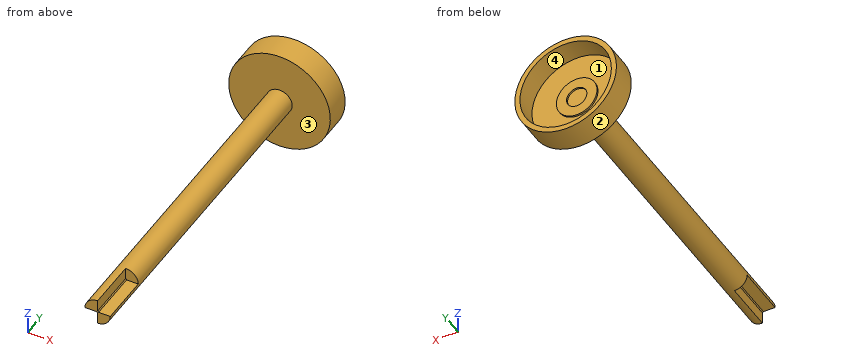
```python
from build123d import *

# Parameters (mm, degrees)
SKETCH1_R           = 10
SKETCH1_R_2         = 9
BOSS_EXTRUDE1_DEPTH = 4.3
BOSS_EXTRUDE2_START = -1
SKETCH1_2_R         = 10
BOSS_EXTRUDE2_DEPTH = 1
SKETCH2_R           = 4
SKETCH2_R_2         = 2
EXTRUDE_THIN1_DEPTH = 0.35
SKETCH3_R           = 2.5
BOSS_EXTRUDE3_DEPTH = 65
CUT_EXTRUDE1_START  = -10
CUT_EXTRUDE1_DEPTH  = 10


with BuildPart() as part:
    # Sketch1 → Boss-Extrude1 (new body)
    with BuildSketch(Plane(origin=(0, 0, 0), x_dir=(1, 0, 0), z_dir=(0, 1, 0))):
        with Locations(Location((0, 0, 0), (0, 0, 90))):
            Circle(SKETCH1_R)
        with Locations(Location((0, 0, 0), (0, 0, 90))):
            Circle(SKETCH1_R_2, mode=Mode.SUBTRACT)
    extrude(amount=BOSS_EXTRUDE1_DEPTH)

    # Sketch1_2 → Boss-Extrude2 (add)
    with BuildSketch(Plane(origin=(0, 0, 0), x_dir=(1, 0, 0), z_dir=(0, 1, 0)).offset(BOSS_EXTRUDE2_START)):
        with Locations(Location((0, 0, 0), (0, 0, 90))):
            Circle(SKETCH1_2_R)
    extrude(amount=BOSS_EXTRUDE2_DEPTH)

    # Sketch2 → Extrude-Thin1 (add)
    with BuildSketch(Plane(origin=(0, 0, 0), x_dir=(1, 0, 0), z_dir=(0, 1, 0))):
        Circle(SKETCH2_R)
        Circle(SKETCH2_R_2, mode=Mode.SUBTRACT)
    extrude(amount=EXTRUDE_THIN1_DEPTH)

    # Sketch3 → Boss-Extrude3 (add)
    with BuildSketch(Plane.XZ.offset(1)):
        with Locations(Location((0, 0, 0), (0, 0, 270))):
            Circle(SKETCH3_R)
    extrude(amount=BOSS_EXTRUDE3_DEPTH)

    # Sketch4 → Cut-Extrude1 (cut)
    with BuildSketch(Plane.XZ.offset(66).offset(CUT_EXTRUDE1_START)):
        with BuildLine():
            Line((-2.5, 0), (-0.194982329, 0))
            ThreePointArc((-0.194982329, 0), (-0.137873327, -0.137873327), (0, -0.194982329))
            Line((0, -0.194982329), (0, -2.5))
            ThreePointArc((0, -2.5), (-1.767766953, -1.767766953), (-2.5, 0))
        make_face()
        with BuildLine():
            Line((0, 2.5), (0, 0.194982329))
            ThreePointArc((0, 0.194982329), (0.137873327, 0.137873327), (0.194982329, 0))
            Line((0.194982329, 0), (2.5, 0))
            ThreePointArc((2.5, 0), (1.767766953, 1.767766953), (0, 2.5))
        make_face()
    extrude(amount=CUT_EXTRUDE1_DEPTH, mode=Mode.SUBTRACT)


solid = part.part
```
For this review, take the finished solid that the model builds, in its own axes (mm). Face numbers are marked on the shaded views. Coordinates: 2 decimals unless noted, no trailing zeros. Loops run counter-clockwise (first coordinate to the right, second up) from the corner with the lowest first, then second, coordinate; pieces in that order, holes last. Notation, with made-up numbers: (-11, -28.75) - (5, -28.75) arc R18 cw to (5, -22.75) - close; hole circle Ø2 at (73.5, 85). An arc over 180 degrees is marked (long way). Use one line per item in the form item = value. Start each with the question number.
1) To check wall thickness, follow probe 1 along X at (y, z) = (0.2, 0); probe 2 along X at (y, z) = (1.55, 0); probe 3 along Y at (x, z) = (2.5, -5.75). State the ranges of each line that lie inside material, in increasing order. Write a range as from..to.
2) For pin 1 (1.2 mm diameter, centred on y = -63.5, z = -1, fed in from -X); pin 2 (12 mm diameter, centred on y = -7.5, z = 3, fed in from -X); pin 3 (0.7 mm diameter, centred on x = -2, y = -61.5, fed in from -Z), all flat-tipped, find the tip position at first contact; note any pin that passes through.
3) Take a section at B-B (z = 7.25). State the section outline as (x, y) points, plus the area to 3 significant figures.
4) Take a section at C-C (y = -46.5). State the section outline as (x, z) points, plus the area to 3 significant figures.
5) Take a section at A-A (y = -57.5). State the section outline as (x, z) points, plus the area to 3 significant figures.
6) Draft analysis for pull direction X (two halves, no side actions). For the marked faces 1, 2, 3 and 4, state which applies: released by +X, released by -X, zero draft, split by the parting line, or undercut.
From the geometry:
q1.probe_1 = -10..-9, -4..-2, 2..4, 9..10
q1.probe_2 = -10..-9, 9..10
q1.probe_3 = -1..0
q2.pin_1 = 0
q2.pin_2 = -2.5
q2.pin_3 = 0
q3.outline = (-6.89, -1) - (6.89, -1) - (6.89, 4.3) - (5.33, 4.3) - (5.33, 0) - (-5.33, 0) - (-5.33, 4.3) - (-6.89, 4.3) - close
q3.area = 27.1 mm2
q4.outline = circle Ø5 at (0, 0)
q4.area = 19.6 mm2
q5.outline = (-2.5, 0) - (-0.19, 0) arc R0.19 ccw to (0, -0.19) - (0, -2.5) arc R2.5 ccw to (2.5, 0) - (0.19, 0) arc R0.19 ccw to (0, 0.19) - (0, 2.5) arc R2.5 ccw to start
q5.area = 9.88 mm2
q6.face_1 = undercut
q6.face_2 = split by the parting line
q6.face_3 = zero draft
q6.face_4 = undercut
